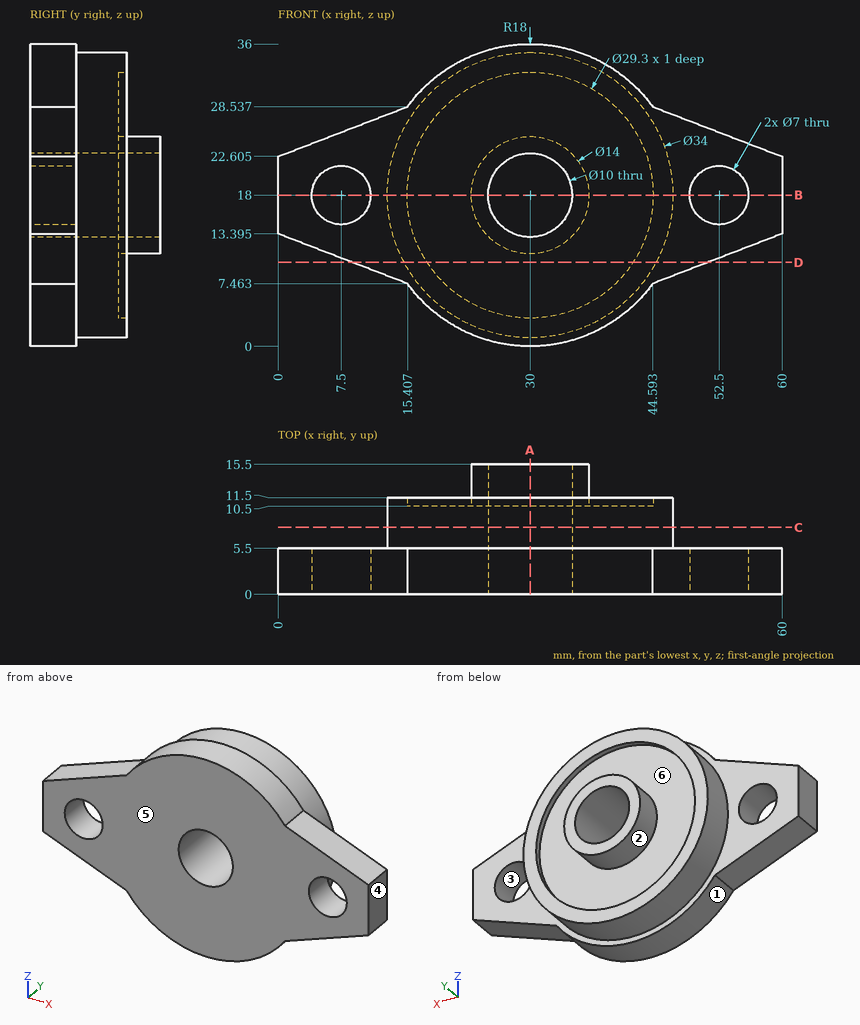
Can you work these out from the drawing? Everything is in mm from the part's minimum corner. A direction names the side the tool comes from. Round coordinates to 2 decimals unless told otherwise and drop trailing zeros. Loops run counter-clockwise (first coordinate to the right, second up) from the corner with the lowest first, then second, coordinate; pieces in that order, holes last. Notation, with made-up numbers: (44, 24) - (84, 24) arc R25 cw to (84, 36) - close; hole circle Ø6 at (30, 84). An arc over 180 degrees is marked (long way). Answer in a Markdown table with one row per item. Add a question column.
(1) If we section it at D-D (z = 10): Please give me the cut outline in (x, y).
(2) If we section it at C-C (y = 8): Please give me the cut outline in (x, z).
(3) If we section it at B-B (z = 18): Please give me the cut outline in (x, y), plus the area to 3 significant figures.
(4) If we mould it in two halves opening along X, with no side actions, what happens to the marked faces 1, 2, 3 and 4? For each: pulls with the +X half, pulls with the -X half, needs draft (parallel to the pull), parting line crosses it, or undercut.
(5) If we section it at A-A (x = 30): Please give me the cut outline in (y, z), plus the area to 3 significant figures.
(6) I'm going to push flat-ended pins straight in: pin 1 (2 mm diameter, centred on x = 32, y = 5, fed in from +Z); pin 2 (8 mm diameter, centred on y = 12, z = 10.5, fed in from -X); pin 3 (9 mm diameter, centred on x = 52.5, z = 18, fed in from +Y). Where does each tip first touch, or does it pass through?
(7) I need wall thicknesses on line 1 along X through (y, z) = (1.65, 18); line 2 along X through (y, z) = (10.9, 18); line 3 along X through (y, z) = (8, 18). Which ranges of each line are inside material? Lowest first, please.
(8) For the marked faces 5 and 6, which set-ups out of +Z, -Z, +X, -X, +Y, -Y let a thin tool reach every point of the face, with its end or its side?
Model answer:
| question | item | result |
|---|---|---|
| 1 | outline | (8.82, 0) - (51.18, 0) - (51.18, 5.5) - (45, 5.5) - (45, 11.5) - (42.27, 11.5) - (42.27, 10.5) - (17.73, 10.5) - (17.73, 11.5) - (15, 11.5) - (15, 5.5) - (8.82, 5.5) - close |
| 2 | outline | circle Ø34 at (30, 18); hole circle Ø10 at (30, 18) |
| 3 | outline | (0, 0) - (4, 0) - (4, 5.5) - (0, 5.5) - close; (11, 0) - (25, 0) - (25, 15.5) - (23, 15.5) - (23, 10.5) - (15.35, 10.5) - (15.35, 11.5) - (13, 11.5) - (13, 5.5) - (11, 5.5) - close; (35, 0) - (49, 0) - (49, 5.5) - (47, 5.5) - (47, 11.5) - (44.65, 11.5) - (44.65, 10.5) - (37, 10.5) - (37, 15.5) - (35, 15.5) - close; (56, 0) - (60, 0) - (60, 5.5) - (56, 5.5) - close |
| 3 | area | 343 mm² |
| 4 | face 1 | parting line crosses it |
| 4 | face 2 | undercut |
| 4 | face 3 | undercut |
| 4 | face 4 | pulls with the +X half |
| 5 | outline | (0, 0) - (5.5, 0) - (5.5, 1) - (11.5, 1) - (11.5, 3.35) - (10.5, 3.35) - (10.5, 11) - (15.5, 11) - (15.5, 13) - (0, 13) - close; (0, 23) - (15.5, 23) - (15.5, 25) - (10.5, 25) - (10.5, 32.65) - (11.5, 32.65) - (11.5, 35) - (5.5, 35) - (5.5, 36) - (0, 36) - close |
| 5 | area | 288 mm² |
| 6 | pin 1 | stops at z = 35.97 |
| 6 | pin 2 | stops at x = 13.37 |
| 6 | pin 3 | stops at y = 5.5 |
| 7 | line 1 | x = 0 to 4, 11 to 25, 35 to 49, 56 to 60 |
| 7 | line 2 | x = 13 to 15.35, 23 to 25, 35 to 37, 44.65 to 47 |
| 7 | line 3 | x = 13 to 25, 35 to 47 |
| 8 | face 5 | +Z, -Z, +X, -X, -Y |
| 8 | face 6 | +Y |
